```python
from build123d import *

# Parameters (mm, degrees)
F2_W        = 22
F2_H        = 42
F2_W_2      = 16
F2_H_2      = 36
F3_DEPTH    = 2
F2_R        = 6
F4_DEPTH    = 25
F5_T1_DEPTH = 14.5024142536
F6_R        = 0.5
F7_R        = 0.2


# Not quite as in the source:
# - a fillet or chamfer that OpenCascade refuses, or shapes differently, is made with other operations: its cross-section is extruded or revolved along the edge and cut away or added


with BuildPart() as f1:
    # F0 (on Right) → F1 (revolve)
    with BuildSketch(Plane.YZ):
        with BuildLine():
            Line((-23, 0), (-21, 0))
            Line((-21, 0), (-21, 32.1))
            Line((-21, 32.1), (-21, 34.1))
            Line((-21, 34.1), (-21, 40))
            ThreePointArc((-21, 40), (-20.1213203436, 42.1213203436), (-18, 43))
            Line((-18, 43), (15, 43))
            Line((15, 43), (17, 43))
            Line((17, 43), (23, 43))
            Line((23, 43), (25, 43))
            Line((25, 43), (25, 45))
            Line((25, 45), (-18, 45))
            ThreePointArc((-18, 45), (-21.5355339059, 43.5355339059), (-23, 40))
            Line((-23, 40), (-23, 0))
        make_face()
    revolve(axis=Axis((0, -22, 0), (0, -1, 0)))

    # F2 (on face) → F3 (join)
    with BuildSketch(Plane(origin=(0, -21, 0), x_dir=(-1, 0, 0), z_dir=(0, 1, 0))):
        Rectangle(F2_W, F2_H)
        Rectangle(F2_W_2, F2_H_2, mode=Mode.SUBTRACT)
    extrude(amount=F3_DEPTH)

    # F2 (on face) → F4 (cut)
    with BuildSketch(Plane(origin=(0, -21, 0), x_dir=(-1, 0, 0), z_dir=(0, 1, 0))):
        Circle(F2_R)
    extrude(amount=-F4_DEPTH, mode=Mode.SUBTRACT)

    # F5: fillet of radius 5 on 4 edges, made by hand

    # F5_s2 → F5_t1 (cut)
    with BuildSketch(Plane.XZ.offset(6.4975857464)):
        with BuildLine():
            ThreePointArc((5.9990343146, 21.0004), (9.5355339059, 19.5355339059), (11.0004, 15.9990343146))
            Line((11.0004, 15.9990343146), (11.5005365685, 15.9990343146))
            ThreePointArc((11.5005365685, 15.9990343146), (11.5001365685, 18.4995171573), (11.5001365685, 21))
            Line((11.5001365685, 21), (11, 21.5001365685))
            ThreePointArc((11, 21.5001365685), (8.4995171573, 21.5001365685), (5.9990343146, 21.5005365685))
            Line((5.9990343146, 21.5005365685), (5.9990343146, 21.0004))
        make_face()
        with BuildLine():
            ThreePointArc((-5.9990343146, 21.0004), (-9.5355339059, 19.5355339059), (-11.0004, 15.9990343146))
            Line((-11.0004, 15.9990343146), (-11.5005365685, 15.9990343146))
            ThreePointArc((-11.5005365685, 15.9990343146), (-11.5001365685, 18.4995171573), (-11.5001365685, 21))
            Line((-11.5001365685, 21), (-11, 21.5001365685))
            ThreePointArc((-11, 21.5001365685), (-8.4995171573, 21.5001365685), (-5.9990343146, 21.5005365685))
            Line((-5.9990343146, 21.5005365685), (-5.9990343146, 21.0004))
        make_face()
        with BuildLine():
            ThreePointArc((-5.9990343146, -21.0004), (-9.5355339059, -19.5355339059), (-11.0004, -15.9990343146))
            Line((-11.0004, -15.9990343146), (-11.5005365685, -15.9990343146))
            ThreePointArc((-11.5005365685, -15.9990343146), (-11.5001365685, -18.4995171573), (-11.5001365685, -21))
            Line((-11.5001365685, -21), (-11, -21.5001365685))
            ThreePointArc((-11, -21.5001365685), (-8.4995171573, -21.5001365685), (-5.9990343146, -21.5005365685))
            Line((-5.9990343146, -21.5005365685), (-5.9990343146, -21.0004))
        make_face()
        with BuildLine():
            ThreePointArc((11.0004, -15.9990343146), (9.5355339059, -19.5355339059), (5.9990343146, -21.0004))
            Line((5.9990343146, -21.0004), (5.9990343146, -21.5005365685))
            ThreePointArc((5.9990343146, -21.5005365685), (8.4995171573, -21.5001365685), (11, -21.5001365685))
            Line((11, -21.5001365685), (11.5001365685, -21))
            ThreePointArc((11.5001365685, -21), (11.5001365685, -18.4995171573), (11.5005365685, -15.9990343146))
            Line((11.5005365685, -15.9990343146), (11.0004, -15.9990343146))
        make_face()
    extrude(amount=F5_T1_DEPTH, mode=Mode.SUBTRACT)

    # F6
    f6_edges = [f1.edges().sort_by_distance(p)[0] for p in [
        (0, -21, -40),
        (0, -21, 21),
        (-9.535534, -21, 19.535534),
        (-11, -21, 0),
        (-9.535534, -21, -19.535534),
        (0, -21, -21),
        (9.535534, -21, -19.535534),
        (11, -21, 0),
        (9.535534, -21, 19.535534),
    ]]
    fillet(f6_edges, radius=F6_R)

    # F7
    f7_edges = [f1.edges().sort_by_distance(p)[0] for p in [
        (8, -21, 0),
        (0, -21, -18),
        (0, -21, 18),
        (-8, -21, 0),
        (6, -21, 0),
        (0, -21, -40),
    ]]
    fillet(f7_edges, radius=F7_R)


solid = f1.part
```
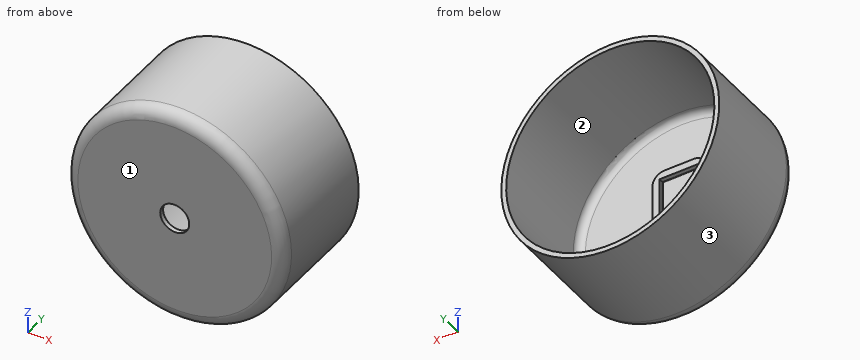
Verification items for the finished model (mm, model axes). Face numbers are marked on the shaded views. Give positions to 0.01 mm unless a question says otherwise; leave off trailing zeros. Order: outer loops, then holes, each group sorted by start corner. A loop starts at its lowest first (then second) coordinate and runs counter-clockwise, first axis right, second up. Notation, with made-up numbers: M -23,34 L 21,34 A18 ccw 21,47 Z; hole C 87.5,32.25 d7. An arc over 180 degrees is marked long. Answer in a Markdown table with one row per item. Add a question column.
Item 1: Gauge pin test, flat ends, axial feed: pin 1 (0.9 mm diameter, centred on x = -2.5, y = -20, fed in from +Z); pin 2 (1.6 mm diameter, centred on x = 2.5, y = -19.5, fed in from -Z); pin 3 (1.6 mm diameter, centred on y = -19.5, z = 7.5, fed in from -X). Record the tip position at first contact, or that the pin passes through.
Item 2: Scan lines: probe 1 along Z at (x, y) = (0, 15); probe 2 along Y at (x, z) = (8.5, 10); probe 3 along X at (y, z) = (-20, 27). Record each from-to range of solid material in increasing order. Write a range as from..to.
Item 3: Section check C-C, the plane y = -10. Enter the section's corners in (x, z).
Item 4: Mould release check, pull along Z, two halves, no side actions. Record for the marked faces 1, 2 and 3: released by +Z, released by -Z, zero draft, split by the parting line, or undercut.
Filled sheet:
| question | item | result |
|---|---|---|
| 1 | pin 1 | stops at z = 44.69 |
| 1 | pin 2 | stops at z = -44.89 |
| 1 | pin 3 | stops at x = -44.37 |
| 2 | probe 1 | z = -45..-43, 43..45 |
| 2 | probe 2 | y = -23..-19 |
| 2 | probe 3 | x = -35.48..-32.48, 32.48..35.48 |
| 3 | outline | C 0,0 d90; hole C 0,0 d86 |
| 4 | face 1 | zero draft |
| 4 | face 2 | undercut |
| 4 | face 3 | split by the parting line |
